Autodesk Fusion 360 part; units mm, degrees
sketch "Boceto1" plane through (0, 0, 0) normal (0, 1, 0) x (1, 0, 0)
  line L0 (-63, -5) -> (67.4, -5)
  line L1 (67.4, 5) -> (-63, 5)
  line L2 (-67.4, 0) -> (67.4, 0) construction
  circle A0 centre (67.4, 0) radius 2.75
  circle A1 centre (-63, 0) radius 2.75
  arc A2 (-63, 5) -> (-63.25, 4.9937) centre (-63, 0) ccw
  arc A3 (-63.25, -4.9937) -> (-63, -5) centre (-63, 0) ccw
  arc A4 (-63.25, 4.9937) -> (-63.25, -4.9937) centre (-63.5, 0) ccw
  arc A5 (67.4, -5) -> (67.65, -4.9937) centre (67.4, 0) ccw
  arc A6 (67.65, 4.9937) -> (67.4, 5) centre (67.4, 0) ccw
  arc A7 (67.65, -4.9937) -> (67.65, 4.9937) centre (67.9, 0) ccw
  dimension "d1" = 10
  dimension "d4" = 5.5
  dimension "d11" = 5.5
  dimension "d12" = 130.4
  dimension "d13" = 10
  dimension "d14" = 0.5
  dimension "d15" = 10
  dimension "d16" = 0.5
extrude "Extruir1" add sketch "Boceto1" along normal blind 5
sketch "Boceto2" plane through (0, 5, 0) normal (0, 1, 0) x (-1, 0, 0)
  circle A0 centre (-67.4, 0) radius 2.75
  line L0 (63, 5) -> (-67.4, 5)
  arc A1 (-67.65, -4.9937) -> (-67.4, -5) centre (-67.4, 0) ccw
  line L1 (-67.4, -5) -> (63, -5)
  circle A2 centre (47.4, 0) radius 2.75
  line L2 (0, 0) -> (0, -16) construction
  circle A3 centre (-47.4, 0) radius 2.75
  arc A4 (-67.65, 4.9937) -> (-67.65, -4.9937) centre (-67.9, 0) ccw
  arc A5 (63, -5) -> (63.25, -4.9937) centre (63, 0) ccw
  arc A6 (63.25, -4.9937) -> (63.25, 4.9937) centre (63.5, 0) ccw
  arc A7 (63.25, 4.9937) -> (63, 5) centre (63, 0) ccw
  arc A8 (-67.4, 5) -> (-67.65, 4.9937) centre (-67.4, 0) ccw
  circle A9 centre (63, 0) radius 2.75
  dimension "d7" = 5.5
  dimension "d17" = 47.4
  dimension "d18" = 47.4
extrude "Extruir2" cut sketch "Boceto2" against normal blind 13 contours A2 | A3
Can you work these out from the model? Positions are in its coordinate system, mm. Round coordinates to 2 decimals unless told otherwise and drop trailing zeros. Loops run counter-clockwise (first coordinate to the right, second up) from the corner with the lowest first, then second, coordinate; pieces in that order, holes last. Notation, with made-up numbers: (15.5, -6.75) - (47.5, -6.75) arc R32 ccw to (47.5, 23.25) - close; hole circle Ø7 at (11, 58). An arc over 180 degrees is marked (long way). Write item = value, one per line. Start each with the question number.
(1) For P1, Ø1.5, axis at y = 1, z = 1.5, coming from the -X side, with a flat end and sliding along its axis, tell me the tip position at first contact or that it passes through.
(2) If I drill on probe 1 along Z at (x, y) = (47.4, 2.8); probe 2 along X at (y, z) = (0.75, -0.5); probe 3 along X at (y, z) = (2.05, 2), over which ranges is the centre line in solid material (lowest first)? Write a range as [from, to].
(3) If we section it at A-A (x = 47.4): Please give me the cut outline in (y, z).
(4) If we mould it in two halves opening along Z, with no side actions, what happens to faces 1 (the face through (72.9, 2.5, -0.1)), 2 (the face through (3, 2, -5)), 3 (the face through (-49.94, 2.54, -1.05))? For each: released by +Z, released by -Z, zero draft, split by the parting line, or undercut.
(5) If we section it at D-D (x = -46.5): Please give me the cut outline in (y, z), and give its area (3 significant figures).
(6) If we section it at C-C (y = 2.3): Please give me the cut outline in (x, z), and give its area (3 significant figures).
(7) If we section it at B-B (z = 0): Please give me the cut outline in (x, y), and give its area (3 significant figures).
Ans:
q1.P1 = -68.44
q2.probe_1 = [-5, -2.75], [2.75, 5]
q2.probe_2 = [-68.47, -65.7], [-60.3, -50.1], [-44.7, 44.7], [50.1, 64.7], [70.1, 72.87]
q2.probe_3 = [-68.08, -64.89], [-61.11, -49.29], [-45.51, 45.51], [49.29, 65.51], [69.29, 72.48]
q3.outline = (0, -5) - (5, -5) - (5, -2.75) - (0, -2.75) - close; (0, 2.75) - (5, 2.75) - (5, 5) - (0, 5) - close
q4.face_1 = split by the parting line
q4.face_2 = released by -Z
q4.face_3 = undercut
q5.outline = (0, -5) - (5, -5) - (5, -2.6) - (0, -2.6) - close; (0, 2.6) - (5, 2.6) - (5, 5) - (0, 5) - close
q5.area = 24.0 mm²
q6.outline = (-63.25, -4.99) arc R5 ccw to (-63, -5) - (67.4, -5) arc R5 ccw to (67.65, -4.99) arc R5 ccw (long way) to (67.65, 4.99) arc R5 ccw to (67.4, 5) - (-63, 5) arc R5 ccw to (-63.25, 4.99) arc R5 ccw (long way) to start; hole circle Ø5.5 at (-63, 0); hole circle Ø5.5 at (-47.4, 0); hole circle Ø5.5 at (47.4, 0); hole circle Ø5.5 at (67.4, 0)
q6.area = 1,300 mm²
q7.outline = (-68.5, 0) - (-65.75, 0) - (-65.75, 5) - (-68.5, 5) - close; (-60.25, 0) - (-50.15, 0) - (-50.15, 5) - (-60.25, 5) - close; (-44.65, 0) - (44.65, 0) - (44.65, 5) - (-44.65, 5) - close; (50.15, 0) - (64.65, 0) - (64.65, 5) - (50.15, 5) - close; (70.15, 0) - (72.9, 0) - (72.9, 5) - (70.15, 5) - close
q7.area = 597 mm²
